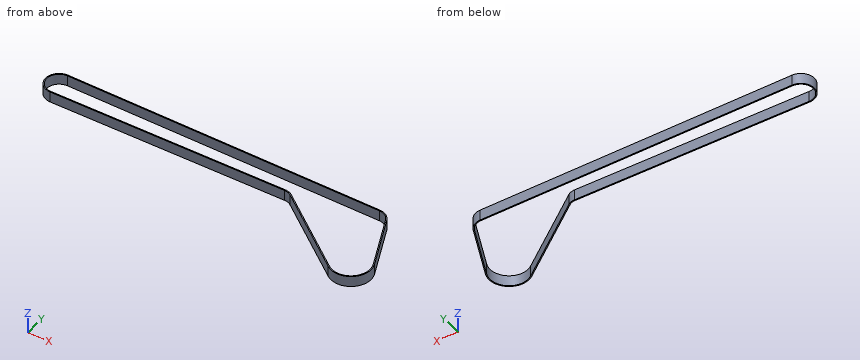
```python
from build123d import *

# Parameters (mm, degrees)
SKETCH_4_W = 10
SKETCH_4_H = 1


with BuildPart() as part:
    # 掃出1: sweep along a path in 草圖2
    with BuildLine(Plane.XY) as sweep_1_path:
        Line((152.003384949, -38.242833415), (130.05681925, 12.006884535))
        ThreePointArc((130.05681925, 12.006884535), (125.863591091, 17.005534481), (119.631157887, 18.935933413))
        Line((119.631157887, 18.935933413), (-175.339326769, 23.108843899))
        ThreePointArc((-175.339326769, 23.108843899), (-187.057488522, 11.636727435), (-175.502777551, 0))
        Line((-175.502777551, 0), (44.192301821, 0))
        ThreePointArc((44.192301821, 0), (47.930804214, -0.621490735), (51.267152631, -2.419108636))
        Line((51.267152631, -2.419108636), (124.846283962, -59.398921136))
        ThreePointArc((124.846283962, -59.398921136), (146.640920811, -59.367491082), (152.003384949, -38.242833415))
    # 草圖4 → 掃出1 (sweep)
    with BuildSketch(Plane(origin=(0, 0, 0), x_dir=(0, 0, -1), z_dir=(1, 0, 0))):
        with Locations((0, -0.5)):
            Rectangle(SKETCH_4_W, SKETCH_4_H)
    sweep(path=sweep_1_path.line)


solid = part.part
```
Check sheet for the modelled part. Datum: model origin and axes. Units: mm. Give positions to 0.01 mm unless a question says otherwise; leave off trailing zeros. Write each loop counter-clockwise with the first axis right and the second up, starting at its lowest first coordinate (ties: lowest second). Pieces come first, ordered by that corner, then holes. Notation, with made-up numbers: (33.25, 53.5) - (83.25, 53.5) arc R17 ccw to (83.25, 73.5) - close; hole circle Ø1 at (80, 54.25). An arc over 180 degrees is marked (long way). Answer as a JSON object with one key per item and string values. Group by question number.
1) Sectioned sample at A-A (z = 2.75). Record the cut outline in (x, y) (3 decimals).
2) Sectioned sample at C-C (y = -12). Record the cut outline in (x, z), then the cut area to 3 significant figures.
3) Sectioned sample at B-B (x = 63). Record the cut outline in (y, z).
4) Depth check by flat-ended pin: P1, Ø5, axis at x = -28, z = -2, coming from the -Y side; P2, Ø5, axis at x = -71.5, z = -2.5, coming from the +Y side; P3, Ø6, axis at y = 4.5, z = -2, coming from the -X side. Enter the tip coordinate at first touch or a pass-through.
5) Thickness scan on probe 1 along Y at (x, z) = (-174, 0); probe 2 along X at (y, z) = (-10.5, 2.5); probe 3 along Y at (x, z) = (-64, -3.5). Record the ranges inside material, lowest first. Write a range as from..to.
Geometry results:
{
 "1": {"outline": "(-175.503, -1) - (44.192, -1) arc R10.555 cw to (50.655, -3.21) - (124.234, -60.19) arc R18.765 ccw to (152.92, -37.843) - (130.973, 12.407) arc R12.555 ccw to (119.645, 19.936) - (-175.325, 24.109) arc R12.555 ccw (long way) to start; hole (-175.503, 0) - (44.192, 0) arc R11.555 cw to (51.267, -2.419) - (124.846, -59.399) arc R17.765 ccw to (152.003, -38.243) - (130.057, 12.007) arc R11.555 ccw to (119.631, 18.936) - (-175.339, 23.109) arc R11.555 ccw (long way) to start"},
 "2": {"outline": "(62.01, -5) - (63.64, -5) - (63.64, 5) - (62.01, 5) - close; (140.54, -5) - (141.63, -5) - (141.63, 5) - (140.54, 5) - close", "area": "27.2 mm^2"},
 "3": {"outline": "(-12.77, -5) - (-11.51, -5) - (-11.51, 5) - (-12.77, 5) - close; (19.74, -5) - (20.74, -5) - (20.74, 5) - (19.74, 5) - close"},
 "4": {"P1": "stops at y = -1", "P2": "stops at y = 22.68", "P3": "stops at x = -187.38"},
 "5": {"probe 1": "y = -1..0, 23.09..24.09", "probe 2": "x = 60.07..61.7, 139.89..140.98", "probe 3": "y = -1..0, 21.53..22.53"}
}
